Could you check a few things on this drawing? It's one solid part, dimensions in mm from its lowest x, y, z. A direction names the side the tool comes from. Coordinates: 2 decimals unless noted, no trailing zeros. Order: outer loops, then holes, each group sorted by start corner. A loop starts at its lowest first (then second) coordinate and runs counter-clockwise, first axis right, second up. Notation, with made-up numbers: (15, 26.5) - (35, 26.5) arc R8 ccw to (35, 40.5) - close; hole circle Ø5 at (40.5, 38). An arc over 180 degrees is marked (long way). Answer in a Markdown table with one row per item. Add a question column.
Item 1: I want a section at D-D (z = 7.5). Please give me the cut outline in (x, y), plus the area to 3 significant figures.
Item 2: Will these pins go through, and if not, where does the flat tip stop? pin 1 Ø2.5 at (x, y) = (9.5, 24) entering from +Z; pin 2 Ø3 at (x, y) = (36, 14.9) entering from -Z; pin 3 Ø4.5 at (x, y) = (16, 14.9) entering from +Z.
Item 3: Thinking about a two-plate mould opening in Y: for the marked faces 3, 4 and 5, which applies, +Y half, -Y half, draft (parallel to the pull), parting line (faces both ways), or undercut?
Item 4: I want a section at C-C (y = 14.9). Please give me the cut outline in (x, z).
Item 5: If I drill on line 1 along Y through (x, z) = (44.24, 5.05); line 2 along Y through (x, z) = (8.53, 5.4); line 3 along X through (y, z) = (14.9, 1.65), over which ranges is the centre line in solid material (lowest first)? Write a range as from..to.
Item 6: On a 3-axis mill with a long thin cutter (end or side, diameter ignored), from which of +Z, -Z, +X, -X, +Y, -Y can I reach the whole of each face in a straight line? I mean the marked faces 1 and 2. Say none if no direction works.
Item 7: I want a section at B-B (x = 16). Please give me the cut outline in (y, z).
Item 8: I want a section at A-A (z = 2.5). Please give me the cut outline in (x, y), plus the area to 3 significant figures.
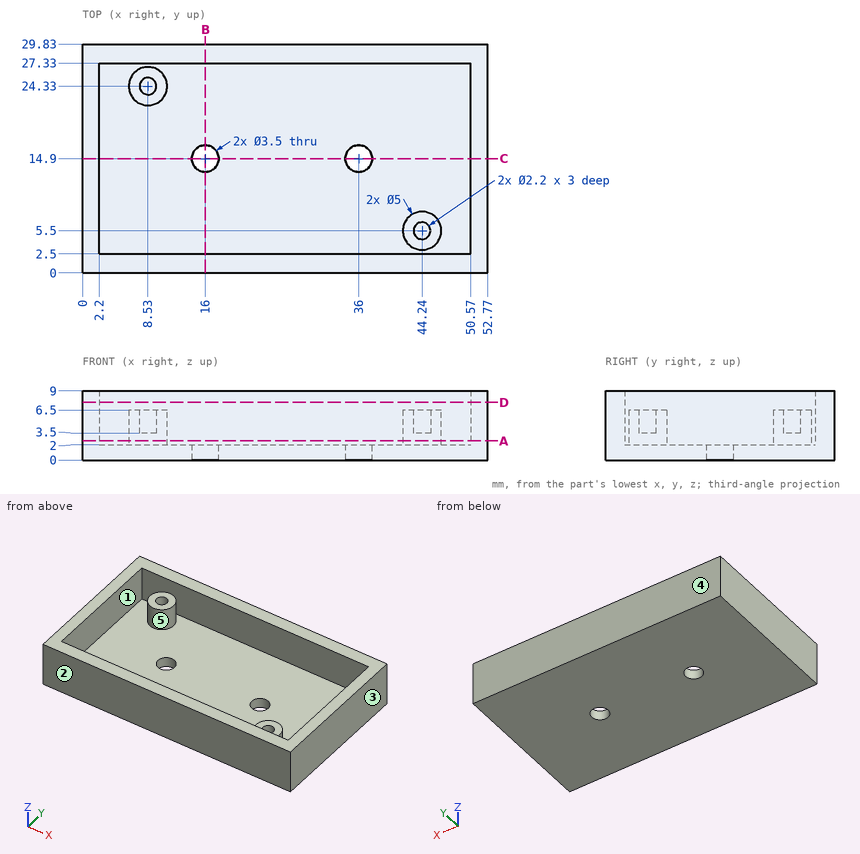
Values follow:
| question | item | result |
|---|---|---|
| 1 | outline | (0, 0) - (52.77, 0) - (52.77, 29.83) - (0, 29.83) - close; hole (2.2, 2.5) - (50.57, 2.5) - (50.57, 27.33) - (2.2, 27.33) - close |
| 1 | area | 373 mm^2 |
| 2 | pin 1 | stops at z = 6.5 |
| 2 | pin 2 | passes through |
| 2 | pin 3 | stops at z = 2 |
| 3 | face 3 | draft |
| 3 | face 4 | +Y half |
| 3 | face 5 | undercut |
| 4 | outline | (0, 0) - (14.25, 0) - (14.25, 2) - (2.2, 2) - (2.2, 9) - (0, 9) - close; (17.75, 0) - (34.25, 0) - (34.25, 2) - (17.75, 2) - close; (37.75, 0) - (52.77, 0) - (52.77, 9) - (50.57, 9) - (50.57, 2) - (37.75, 2) - close |
| 5 | line 1 | y = 0..2.5, 3..4.4, 6.6..8, 27.33..29.83 |
| 5 | line 2 | y = 0..2.5, 21.83..23.23, 25.43..26.83, 27.33..29.83 |
| 5 | line 3 | x = 0..14.25, 17.75..34.25, 37.75..52.77 |
| 6 | face 1 | +Z |
| 6 | face 2 | +Z, -Z, +X, -X, -Y |
| 7 | outline | (0, 0) - (13.15, 0) - (13.15, 2) - (2.5, 2) - (2.5, 9) - (0, 9) - close; (16.65, 0) - (29.83, 0) - (29.83, 9) - (27.33, 9) - (27.33, 2) - (16.65, 2) - close |
| 8 | outline | (0, 0) - (52.77, 0) - (52.77, 29.83) - (0, 29.83) - close; circle Ø5 at (8.53, 24.33); circle Ø5 at (44.24, 5.5); hole (2.2, 2.5) - (50.57, 2.5) - (50.57, 27.33) - (2.2, 27.33) - close |
| 8 | area | 412 mm^2 |
